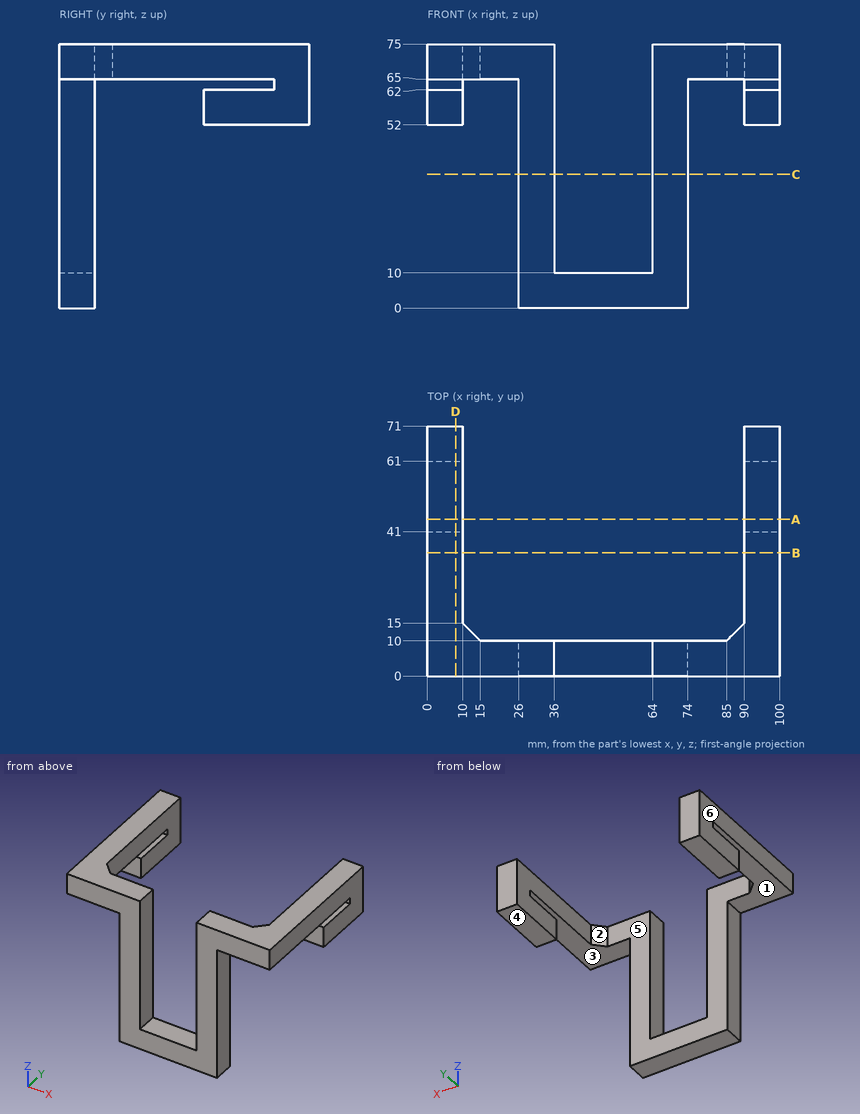
The drawing under review shows one solid part. Ordinate dimensions are in mm from its lowest x, y, z. A direction names the side the tool comes from. Round coordinates to 2 decimals unless told otherwise and drop trailing zeros. Loops run counter-clockwise (first coordinate to the right, second up) from the corner with the lowest first, then second, coordinate; pieces in that order, holes last. Notation, with made-up numbers: (71.25, 56) - (75.25, 56) arc R35 cw to (75.25, 92) - close; hole circle Ø11 at (58.5, 73). An arc over 180 degrees is marked (long way). One line per question, with ' | ' between items.
Q1. Take a section at D-D (x = 8). Give the boundary of the cut face in (y, z), and give its area (3 significant figures).
Taken from the geometry:
outline: (0, 65) - (61, 65) - (61, 62) - (41, 62) - (41, 52) - (71, 52) - (71, 75) - (0, 75) - close | area: 1,040 mm²
Q2. Take a section at B-B (y = 35). Give the boundary of the cut face in (x, z), and give its area (3 significant figures).
Taken from the geometry:
outline: (0, 65) - (10, 65) - (10, 75) - (0, 75) - close; (90, 65) - (100, 65) - (100, 75) - (90, 75) - close | area: 200 mm²
Q3. Tool access review of the marked faces 5 and 6: name each direction out of +Z, -Z, +X, -X, +Y, -Y from which nothing blocks a thin tool from reaching the whole face with its end or side.
Taken from the geometry:
face 5: +Z, -Z, +Y | face 6: +Z, -Z, -X, +Y, -Y
Q4. For line 1 along X through (y, z) = (35, 72.5); line 2 along Y through (x, z) = (73, 46.5); line 3 along Z through (x, y) = (96, 68), list the stretches that pass through material, from the lowest coordinate up. Write a range as [from, to].
Taken from the geometry:
line 1: x = [0, 10], [90, 100] | line 2: y = [0, 10] | line 3: z = [52, 75]
Q5. Take a section at C-C (z = 38). Give the boundary of the cut face in (x, y), and give its area (3 significant figures).
Taken from the geometry:
outline: (26, 0) - (36, 0) - (36, 10) - (26, 10) - close; (64, 0) - (74, 0) - (74, 10) - (64, 10) - close | area: 200 mm²
Q6. The part is to be moulded in two halves that separate along Z. For the marked faces 1, 2, 3 and 4, say which applies: released by +Z, released by -Z, zero draft, split by the parting line, or undercut.
Taken from the geometry:
face 1: undercut | face 2: zero draft | face 3: undercut | face 4: released by -Z
Q7. Take a section at A-A (y = 44.5). Give the boundary of the cut face in (x, z), and give its area (3 significant figures).
Taken from the geometry:
outline: (0, 52) - (10, 52) - (10, 62) - (0, 62) - close; (0, 65) - (10, 65) - (10, 75) - (0, 75) - close; (90, 52) - (100, 52) - (100, 62) - (90, 62) - close; (90, 65) - (100, 65) - (100, 75) - (90, 75) - close | area: 400 mm²
Q8. For pin 1 (11 mm diameter, centred on x = 7, y = 63, fed in from -Z); pin 2 (8 mm diameter, centred on x = 31, y = 10.5, fed in from +Z); pin 3 (3 mm diameter, centred on y = 5, z = 18.5, fed in from -X); pin 4 (8 mm diameter, centred on x = 13, y = 30, fed in from -Z), all flat-tipped, find the tip position at first contact; note any pin that passes through.
Taken from the geometry:
pin 1: stops at z = 52 | pin 2: stops at z = 75 | pin 3: stops at x = 26 | pin 4: stops at z = 65
